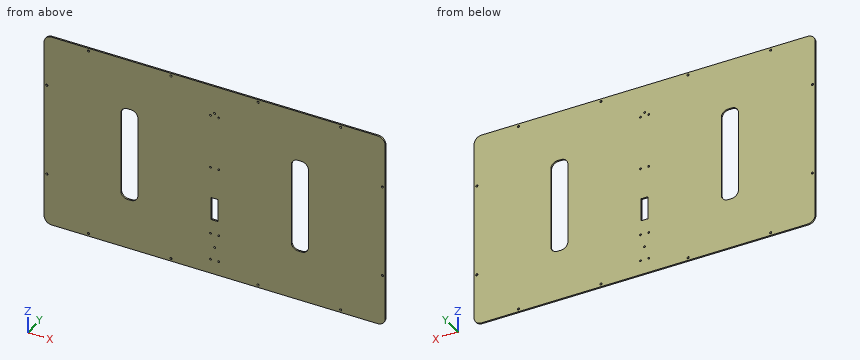
from build123d import *

# Parameters (mm, degrees)
SKETCH1_R           = 1.6
SKETCH1_R_2         = 1.4
SKETCH1_W           = 10
SKETCH1_H           = 34
BOSS_EXTRUDE1_DEPTH = 2.2
SKETCH2_R           = 1.35
CUT_EXTRUDE1_DEPTH  = 59.2


with BuildPart() as part:
    # Sketch1 → Boss-Extrude1 (new body)
    with BuildSketch(Plane(origin=(0, 0, 0), x_dir=(1, 0, 0), z_dir=(0, 1, 0))):
        with BuildLine():
            Line((-239, 145), (239, 145))
            ThreePointArc((239, 145), (246.778174593, 141.778174593), (250, 134))
            Line((250, 134), (250, -134))
            ThreePointArc((250, -134), (246.778174593, -141.778174593), (239, -145))
            Line((239, -145), (-239, -145))
            ThreePointArc((-239, -145), (-246.778174593, -141.778174593), (-250, -134))
            Line((-250, -134), (-250, 134))
            ThreePointArc((-250, 134), (-246.778174593, 141.778174593), (-239, 145))
        make_face()
        with Locations(Location((63.75, 141, 0), (0, 0, 270))):
            Circle(SKETCH1_R, mode=Mode.SUBTRACT)
        with Locations(Location((184.75, 141, 0), (0, 0, 270))):
            Circle(SKETCH1_R, mode=Mode.SUBTRACT)
        with Locations(Location((246, 68.5, 0), (0, 0, 270))):
            Circle(SKETCH1_R, mode=Mode.SUBTRACT)
        with Locations(Location((0, 103.5, 0), (0, 0, 270))):
            Circle(SKETCH1_R_2, mode=Mode.SUBTRACT)
        with Locations(Location((0, -103.5, 0), (0, 0, 270))):
            Circle(SKETCH1_R_2, mode=Mode.SUBTRACT)
        with Locations(Location((-246, 68.5, 0), (0, 0, 90))):
            Circle(SKETCH1_R, mode=Mode.SUBTRACT)
        with Locations(Location((-184.75, 141, 0), (0, 0, 90))):
            Circle(SKETCH1_R, mode=Mode.SUBTRACT)
        with Locations(Location((-63.75, 141, 0), (0, 0, 90))):
            Circle(SKETCH1_R, mode=Mode.SUBTRACT)
        with Locations(Location((184.75, -141, 0), (0, 0, 90))):
            Circle(SKETCH1_R, mode=Mode.SUBTRACT)
        with Locations(Location((246, -68.5, 0), (0, 0, 90))):
            Circle(SKETCH1_R, mode=Mode.SUBTRACT)
        with Locations(Location((63.75, -141, 0), (0, 0, 90))):
            Circle(SKETCH1_R, mode=Mode.SUBTRACT)
        with Locations(Location((-63.75, -141, 0), (0, 0, 270))):
            Circle(SKETCH1_R, mode=Mode.SUBTRACT)
        with Locations(Location((-184.75, -141, 0), (0, 0, 270))):
            Circle(SKETCH1_R, mode=Mode.SUBTRACT)
        with Locations(Location((-246, -68.5, 0), (0, 0, 270))):
            Circle(SKETCH1_R, mode=Mode.SUBTRACT)
        with BuildLine():
            Line((-127.5, -70), (-122.5, -70))
            ThreePointArc((-122.5, -70), (-115.428932188, -67.071067812), (-112.5, -60))
            Line((-112.5, -60), (-112.5, 60))
            ThreePointArc((-112.5, 60), (-115.428932188, 67.071067812), (-122.5, 70))
            Line((-122.5, 70), (-127.5, 70))
            ThreePointArc((-127.5, 70), (-134.571067812, 67.071067812), (-137.5, 60))
            Line((-137.5, 60), (-137.5, -60))
            ThreePointArc((-137.5, -60), (-134.571067812, -67.071067812), (-127.5, -70))
        make_face(mode=Mode.SUBTRACT)
        with BuildLine():
            Line((122.5, -70), (127.5, -70))
            ThreePointArc((127.5, -70), (134.571067812, -67.071067812), (137.5, -60))
            Line((137.5, -60), (137.5, 60))
            ThreePointArc((137.5, 60), (134.571067812, 67.071067812), (127.5, 70))
            Line((127.5, 70), (122.5, 70))
            ThreePointArc((122.5, 70), (115.428932188, 67.071067812), (112.5, 60))
            Line((112.5, 60), (112.5, -60))
            ThreePointArc((112.5, -60), (115.428932188, -67.071067812), (122.5, -70))
        make_face(mode=Mode.SUBTRACT)
        with Locations((0, 45)):
            Rectangle(SKETCH1_W, SKETCH1_H, mode=Mode.SUBTRACT)
    extrude(amount=BOSS_EXTRUDE1_DEPTH)

    # Sketch2 → Cut-Extrude1 (cut)
    with BuildSketch(Plane(origin=(0, 2.2, 0), x_dir=(1, 0, 0), z_dir=(0, 1, 0))):
        with Locations(Location((-6, -18.5, 0), (0, 0, 270))):
            Circle(SKETCH2_R)
        with Locations(Location((6, -18.5, 0), (0, 0, 270))):
            Circle(SKETCH2_R)
        with Locations(Location((-6, -98.5, 0), (0, 0, 270))):
            Circle(SKETCH2_R)
        with Locations(Location((6, -98.5, 0), (0, 0, 270))):
            Circle(SKETCH2_R)
        with Locations(Location((-6, 123.5, 0), (0, 0, 270))):
            Circle(SKETCH2_R)
        with Locations(Location((6, 123.5, 0), (0, 0, 270))):
            Circle(SKETCH2_R)
        with Locations(Location((-6, 83.5, 0), (0, 0, 270))):
            Circle(SKETCH2_R)
        with Locations(Location((6, 83.5, 0), (0, 0, 270))):
            Circle(SKETCH2_R)
    extrude(amount=-CUT_EXTRUDE1_DEPTH, mode=Mode.SUBTRACT)


solid = part.part
Here's how the part is built. I have some questions about the finished solid (model axes, mm). Coordinates: 2 decimals unless noted, no trailing zeros. Loops run counter-clockwise (first coordinate to the right, second up) from the corner with the lowest first, then second, coordinate; pieces in that order, holes last.
1. Imagine slicing it at B-B, the plane y = 1.3. Count the separate pieces of the cut face and the enclosed holes in it, and give its area (3 significant figures).
2. Imagine slicing it at A-A, the plane z = 31.5. Please give me the cut outline in (x, y), and give its area (3 significant figures).
3. I need wall thicknesses on L1, parallel to X at y = 0.2, z = 42; L2, parallel to X at y = 1, z = -141; L3, parallel to X at y = 1.3, z = 98.5. Which ranges of each line are inside material? Lowest first, please.
4. For P1, Ø2.5, axis at x = -184.75, z = -141, coming from the -Y side, with a flat end and sliding along its axis, tell me the tip position at first contact or that it passes through.
Taken from the geometry:
1. separate pieces: 1
1. enclosed holes: 25
1. area: 138,000 mm2
2. outline: (-250, 0) - (-137.5, 0) - (-137.5, 2.2) - (-250, 2.2) - close; (-112.5, 0) - (112.5, 0) - (112.5, 2.2) - (-112.5, 2.2) - close; (137.5, 0) - (250, 0) - (250, 2.2) - (137.5, 2.2) - close
2. area: 990 mm2
3. L1: x = -250 to -137.5, -112.5 to 112.5, 137.5 to 250
3. L2: x = -247.49 to -186.35, -183.15 to -65.35, -62.15 to 62.15, 65.35 to 183.15, 186.35 to 247.49
3. L3: x = -250 to -7.35, -4.65 to 4.65, 7.35 to 250
4. P1: passes through
